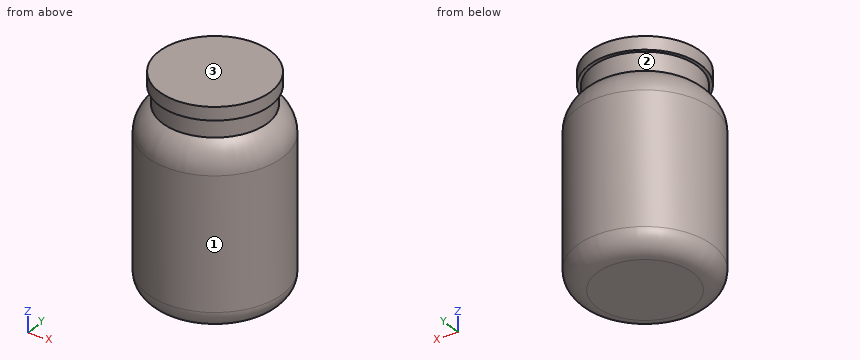
```python
from build123d import *

# Parameters (mm, degrees)
SKETCH_R     = 51.5
PAD_DEPTH    = 140
FILLET_R     = 25
FILLET001_R  = 15
SKETCH001_R  = 40
PAD001_DEPTH = 30
SKETCH002_R  = 42.5
PAD002_DEPTH = 10


with BuildPart() as part:
    # Sketch → Pad (new body)
    with BuildSketch(Plane.XY):
        Circle(SKETCH_R)
    extrude(amount=PAD_DEPTH)

    # Fillet
    fillet_edges = [part.edges().sort_by_distance(p)[0] for p in [
        (-51.5, 0, 140),
    ]]
    fillet(fillet_edges, radius=FILLET_R)

    # Fillet001
    fillet001_edges = [part.edges().sort_by_distance(p)[0] for p in [
        (-51.5, 0, 0),
    ]]
    fillet(fillet001_edges, radius=FILLET001_R)

    # Sketch001 (on Face5 of Fillet001) → Pad001 (join)
    with BuildSketch(Plane.XY.offset(130)):
        Circle(SKETCH001_R)
    extrude(amount=PAD001_DEPTH)

    # Sketch002 (on Face6 of Pad001) → Pad002 (join)
    with BuildSketch(Plane.XY.offset(160)):
        Circle(SKETCH002_R)
    extrude(amount=-PAD002_DEPTH)


solid = part.part
```
Build history of the part. All positions in model axes, mm. Face numbers are marked on the shaded views. Round coordinates to 2 decimals unless told otherwise and drop trailing zeros. Loops run counter-clockwise (first coordinate to the right, second up) from the corner with the lowest first, then second, coordinate; pieces in that order, holes last. Notation, with made-up numbers: M 84,-35.5 L 121,-35.5 A25 cw 121,-2.5 Z; hole C -27.5,5.25 d3. An arc over 180 degrees is marked long. Answer as CSV lines item,"result".
1. Wall check: probe 1 along Z at (x, y) = (-25, -32.5); probe 2 along Z at (x, y) = (12, -45); probe 3 along Y at (x, z) = (-27, 22.5). Give the ranges that are in metal, low to high. Write a range as [from, to].
Resolved:
probe 1,"z = [0.69, 135.36], [150, 160]"
probe 2,"z = [3.88, 129.9]"
probe 3,"y = [-43.85, 43.85]"
2. Cut at A-A on y = 0. Write the cut outline in (x, z).
Resolved:
outline,"M -51.5,15 A15 ccw -36.5,0 L 36.5,0 A15 ccw 51.5,15 L 51.5,115 A25 ccw 40,136.04 L 40,150 L 42.5,150 L 42.5,160 L -42.5,160 L -42.5,150 L -40,150 L -40,136.04 A25 ccw -51.5,115 Z"
3. Cut at D-D on z = 88. Write the cut outline in (x, y).
Resolved:
outline,"C 0,0 d103"
4. Two-plate mould, pull along Z, no slides. Class the marked faces 1, 2 and 3: released by +Z, released by -Z, zero draft, split by the parting line, or undercut.
Resolved:
face 1,"zero draft"
face 2,"undercut"
face 3,"released by +Z"
5. Flat gauge pins, fed straight in: P1, Ø6, axis at y = -23, z = 27.5, coming from the -X side; P2, Ø4, axis at x = 27.5, z = 117, coming from the +Y side; P3, Ø1, axis at y = -16, z = 24.5, coming from the +X side; P4, Ø12, axis at x = -18, y = -5, coming from the -Z side. Where does each tip first touch, or does it go through?
Resolved:
P1,"stops at x = -47.46"
P2,"stops at y = 44.66"
P3,"stops at x = 49.11"
P4,"stops at z = 0"
6. Cut at C-C on z = 122. Write the cut outline in (x, y), then the cut area to 3 significant figures.
Resolved:
outline,"C 0,0 d101"
area,"8,010 mm²"
